Here's how the part is built. I have some questions about the finished solid (model axes, mm). A direction names the side the tool comes from. Coordinates: 2 decimals unless noted, no trailing zeros. Loops run counter-clockwise (first coordinate to the right, second up) from the corner with the lowest first, then second, coordinate; pieces in that order, holes last. Notation, with made-up numbers: M -9,-8.75 L 42,-8.75 A24 ccw 42,25.25 Z; hole C 77,-39 d10. An arc over 180 degrees is marked long. Use one line per item in the form item = value. Start each with the question number.
(1) Imagine slicing it at B-B, the plane z = -2.5. Please give me the cut outline in (x, y), and give its area (3 significant figures).
(2) Will these pins go through, and if not, where does the flat tip stop? P1, Ø3, axis at x = -5.5, z = -3.5, coming from the -Y side; P2, Ø5, axis at x = 8.5, y = 38, coming from the +Z side; P3, Ø1.2, axis at y = 43, z = 1.5, coming from the -X side.
(3) Please list where these lines run through material, in increasing order: L1, parallel to Y at x = 1.75, z = 4.25; L2, parallel to Z at x = -4.5, y = 4; L3, parallel to X at y = 44, z = 2.25.
(4) Thinking about a two-plate mould opening in Y: for faces 4 (the cylindrical face through (13.63, 22.8, -2.46)), 5 (the flat face through (0, 25, 0)), 6 (the flat face through (0, 8.868, 3)), 7 (the flat face through (0, 43, 5.6)), which applies, +Y half, -Y half, draft (parallel to the pull), parting line (faces both ways), or undercut?
(5) Imagine slicing it at A-A, the plane z = 4.5. Please give me the cut outline in (x, y), and give its area (3 significant figures).
(6) Imagine slicing it at D-D, the plane y = 7.5. Please give me the cut outline in (x, z).
(7) On a 3-axis mill with a long thin cutter (end or side, diameter ignored), from which of +Z, -Z, +X, -X, +Y, -Y can I reach the whole of each face in a straight line? I mean faces 1 (the flat face through (0, 4.868, 3)), 2 (the flat face through (0, 44.695, 3)), 3 (the flat face through (-4.75, 7, 3)). Say none if no direction works.
(8) Imagine slicing it at C-C, the plane x = 4. Please give me the cut outline in (y, z).
```python
from build123d import *

# Parameters (mm, degrees)
F1_DEPTH = 5
F3_DEPTH = 5.6


with BuildPart() as f1:
    # F0 (on Top) → F1 (new body)
    with BuildSketch(Plane.XY):
        with BuildLine():
            ThreePointArc((10.507595, 42.815993), (9.425797, 45.734413), (8.107674, 48.55399))
            ThreePointArc((8.107674, 48.55399), (4.748236, 52.508255), (0, 54.600213))
            ThreePointArc((0, 54.600213), (-4.748236, 52.508255), (-8.107674, 48.55399))
            ThreePointArc((-8.107674, 48.55399), (-9.425797, 45.734413), (-10.507595, 42.815993))
            ThreePointArc((-10.507595, 42.815993), (-13.630387, 23.077428), (-10.507595, 3.338862))
            ThreePointArc((-10.507595, 3.338862), (-6.522182, -2.854452), (0, -6.275239))
            ThreePointArc((0, -6.275239), (6.522182, -2.854452), (10.507595, 3.338862))
            ThreePointArc((10.507595, 3.338862), (13.630387, 23.077428), (10.507595, 42.815993))
        make_face()
    extrude(amount=-F1_DEPTH)

    # F2 (on Top) → F3 (join)
    with BuildSketch(Plane.XY):
        Polygon((4.75, 8.868314), (0, 8.868314), (-4.75, 8.868314), (-4.75, 4.868314), (0, 4.868314), (4.75, 4.868314), align=None)
        Polygon((4.75, 44.695161), (0, 44.695161), (-4.75, 44.695161), (-4.75, 40.695161), (0, 40.695161), (4.75, 40.695161), align=None)
    extrude(amount=F3_DEPTH)


solid = f1.part
```
Answer:
q1.outline = M -10.51,3.34 A14.43 ccw 0,-6.28 A14.43 ccw 10.51,3.34 A63.94 ccw 10.51,42.82 A37.82 ccw 8.11,48.55 A11.59 ccw 0,54.6 A11.59 ccw -8.11,48.55 A37.82 ccw -10.51,42.82 A63.94 ccw Z
q1.area = 1,300 mm²
q2.P1 = -4.7
q2.P2 = 0
q2.P3 = -4.75
q3.L1 = 4.87 to 8.87, 40.7 to 44.7
q3.L2 = -5 to 0
q3.L3 = -4.75 to 4.75
q4.face_4 = parting line
q4.face_5 = undercut
q4.face_6 = undercut
q4.face_7 = draft
q5.outline = M -4.75,4.87 L 4.75,4.87 L 4.75,8.87 L -4.75,8.87 Z; M -4.75,40.7 L 4.75,40.7 L 4.75,44.7 L -4.75,44.7 Z
q5.area = 76.0 mm²
q6.outline = M -11.7,-5 L 11.7,-5 L 11.7,0 L 4.75,0 L 4.75,5.6 L -4.75,5.6 L -4.75,0 L -11.7,0 Z
q7.face_1 = +Z, +X, -X, -Y
q7.face_2 = +Z, +X, -X, +Y
q7.face_3 = +Z, -X, +Y, -Y
q8.outline = M -4.7,-5 L 53.02,-5 L 53.02,0 L 44.7,0 L 44.7,5.6 L 40.7,5.6 L 40.7,0 L 8.87,0 L 8.87,5.6 L 4.87,5.6 L 4.87,0 L -4.7,0 Z
